Geometry: final body of the model. Coordinates: model frame, mm. A direction names the side the tool comes from. Coordinates: 2 decimals unless noted, no trailing zeros. Loops run counter-clockwise (first coordinate to the right, second up) from the corner with the lowest first, then second, coordinate; pieces in that order, holes last. Notation, with made-up numbers: (56, -6.75) - (103, -6.75) arc R14 cw to (103, 7.25) - close; hole circle Ø3 at (-24, -20). An arc over 180 degrees is marked (long way). Answer in a Markdown table with one row per item.
from build123d import *

# Parameters (mm, degrees)
SKETCH1_W           = 78
SKETCH1_H           = 40
BOSS_EXTRUDE1_DEPTH = 22
SHELL1_T            = -1.5
SKETCH2_R           = 1.5
CUT_EXTRUDE1_DEPTH  = 50.040799341


with BuildPart() as part:
    # Sketch1 → Boss-Extrude1 (new body)
    with BuildSketch(Plane(origin=(0, 0, 0), x_dir=(1, 0, 0), z_dir=(0, 1, 0))):
        Rectangle(SKETCH1_W, SKETCH1_H)
    extrude(amount=BOSS_EXTRUDE1_DEPTH)

    # Shell1
    shell1_openings = [part.faces().sort_by_distance(p)[0] for p in [
        (0, 22, 0),
    ]]
    offset(amount=SHELL1_T, openings=shell1_openings, kind=Kind.INTERSECTION)

    # Sketch2 → Cut-Extrude1 (cut, through all)
    with BuildSketch(Plane.XZ):
        with Locations(Location((27.5, 9.6, 0), (0, 0, 270))):
            Circle(SKETCH2_R)
        with Locations(Location((27.5, -9.6, 0), (0, 0, 270))):
            Circle(SKETCH2_R)
        with Locations(Location((-27.5, -9.6, 0), (0, 0, 270))):
            Circle(SKETCH2_R)
        with Locations(Location((-27.5, 9.6, 0), (0, 0, 270))):
            Circle(SKETCH2_R)
    extrude(amount=-CUT_EXTRUDE1_DEPTH, mode=Mode.SUBTRACT)


solid = part.part
(1) Cut plane D-D on z = -14.5. Output: boundary loops of the cut face in (x, y).
Verdict:
| item | result |
|---|---|
| outline | (-39, 0) - (39, 0) - (39, 22) - (37.5, 22) - (37.5, 1.5) - (-37.5, 1.5) - (-37.5, 22) - (-39, 22) - close |
(2) Cut plane B-B on z = 9.6. Output: boundary loops of the cut face in (x, y), then the cut area to 4 significant figures.
Verdict:
| item | result |
|---|---|
| outline | (-39, 0) - (-29, 0) - (-29, 1.5) - (-37.5, 1.5) - (-37.5, 22) - (-39, 22) - close; (-26, 0) - (26, 0) - (26, 1.5) - (-26, 1.5) - close; (29, 0) - (39, 0) - (39, 22) - (37.5, 22) - (37.5, 1.5) - (29, 1.5) - close |
| area | 169.5 mm² |
(3) Cut plane C-C on y = 10.75. Output: boundary loops of the cut face in (x, z).
Verdict:
| item | result |
|---|---|
| outline | (-39, -20) - (39, -20) - (39, 20) - (-39, 20) - close; hole (-37.5, -18.5) - (37.5, -18.5) - (37.5, 18.5) - (-37.5, 18.5) - close |
(4) Cut plane A-A on x = -27.5. Output: boundary loops of the cut face in (y, z), then the cut area to 4 significant figures.
Verdict:
| item | result |
|---|---|
| outline | (0, -20) - (22, -20) - (22, -18.5) - (1.5, -18.5) - (1.5, -11.1) - (0, -11.1) - close; (0, -8.1) - (1.5, -8.1) - (1.5, 8.1) - (0, 8.1) - close; (0, 11.1) - (1.5, 11.1) - (1.5, 18.5) - (22, 18.5) - (22, 20) - (0, 20) - close |
| area | 112.5 mm² |
(5) Ray query, probe 1 along X at (y, z) = (0.95, 9.6); probe 2 along Z at (x, y) = (22.5, 13.5); probe 3 along X at (y, z) = (17.5, 7). Return the intervals inside material, ascending.
Verdict:
| item | result |
|---|---|
| probe 1 | x = -39 to -29, -26 to 26, 29 to 39 |
| probe 2 | z = -20 to -18.5, 18.5 to 20 |
| probe 3 | x = -39 to -37.5, 37.5 to 39 |
(6) Pull-direction query (X, two-part tool) for faces 3 (the face through (-39, 11, 0)), 4 (the face through (-12, 22, 19)), 5 (the face through (-37.5, 12, 0)); classes: pulls with the +X half, pulls with the -X half, needs draft (parallel to the pull), parting line crosses it, or undercut.
Verdict:
| item | result |
|---|---|
| face 3 | pulls with the -X half |
| face 4 | needs draft |
| face 5 | undercut |
(7) Access query for faces 1 (the face through (-1, 11, -20)), 2 (the face through (-1, 12, 18.5)). Directions: +Z, -Z, +X, -X, +Y, -Y. A direction counts if a zero-diameter tool reaches every point of the face in a straight line with its end or side. Return the directions, or none.
Verdict:
| item | result |
|---|---|
| face 1 | -Z, +X, -X, +Y, -Y |
| face 2 | +Y |
(8) First-contact query: pin 1 Ø1 at (x, z) = (-2.5, -2) entering from +Y. Flat tip, straight axial feed; report the tip coordinate or a pass-through.
Verdict:
| item | result |
|---|---|
| pin 1 | stops at y = 1.5 |
